from build123d import *

# Parameters (mm, degrees)
SKETCH4_R             = 2.54
SKETCH4_R_2           = 1.8161
BOSS_EXTRUDE1_DEPTH   = 2.38125
BOSS_EXTRUDE1_2_DEPTH = 2.38125
SKETCH5_R             = 1.7907
BOSS_EXTRUDE2_DEPTH   = 1.27


with BuildPart() as part:
    # Sketch4 → Boss-Extrude1 (new, symmetric)
    with BuildSketch(Plane.XY):
        with Locations(Location((-4.7625, 0, 0), (0, 0, 180))):
            Circle(SKETCH4_R)
        with Locations(Location((-4.7625, 0, 0), (0, 0, 180))):
            Circle(SKETCH4_R_2, mode=Mode.SUBTRACT)
    extrude(amount=BOSS_EXTRUDE1_DEPTH, both=True)


with BuildPart() as body_2:
    # Sketch4 → Boss-Extrude1 2 (new, symmetric)
    with BuildSketch(Plane.XY):
        with Locations(Location((4.7625, 0, 0), (0, 0, 180))):
            Circle(SKETCH4_R)
        with Locations(Location((4.7625, 0, 0), (0, 0, 180))):
            Circle(SKETCH4_R_2, mode=Mode.SUBTRACT)
    extrude(amount=BOSS_EXTRUDE1_2_DEPTH, both=True)


with BuildPart() as body_3:
    # Sketch5 → Boss-Extrude2 (new body)
    with BuildSketch(Plane.XY.offset(2.38125)):
        with BuildLine():
            ThreePointArc((-3.562267566, 4.240307738), (-9.1694, 0), (-3.562267566, -4.240307738))
            ThreePointArc((-3.562267566, -4.240307738), (0, -3.745865), (3.562267566, -4.240307738))
            ThreePointArc((3.562267566, -4.240307738), (9.1694, 0), (3.562267566, 4.240307738))
            ThreePointArc((3.562267566, 4.240307738), (0, 3.745865), (-3.562267566, 4.240307738))
        make_face()
        with Locations((-4.7625, 0)):
            Circle(SKETCH5_R, mode=Mode.SUBTRACT)
        with Locations((4.7625, 0)):
            Circle(SKETCH5_R, mode=Mode.SUBTRACT)
    extrude(amount=BOSS_EXTRUDE2_DEPTH)


with BuildPart() as body_4:
    # Mirror3: mirrored copy
    add(body_3.part.mirror(Plane.XY))

    # Combine2: union body 3, body 2, part
    add(body_3.part)
    add(body_2.part)
    add(part.part)


solid = body_4.part
For this review, take the finished solid that the model builds, in its own axes (mm). A direction names the side the tool comes from. Give positions to 0.01 mm unless a question says otherwise; leave off trailing zeros. Loops run counter-clockwise (first coordinate to the right, second up) from the corner with the lowest first, then second, coordinate; pieces in that order, holes last. Notation, with made-up numbers: M 64.5,32.25 L 87.5,32.25 A14 cw 87.5,38.25 Z; hole C -35.5,68 d6. An arc over 180 degrees is marked long. Answer as a JSON object with one key per item and string values. Group by question number.
Q1. Add section A-A on z = 0.75. Give the boundary of the cut face in (x, y), and give its area (3 significant figures).
Q2. Add section C-C on x = -1. Give the boundary of the cut face in (y, z).
Q3. Tool access review of faces 4 (the cylindrical face through (2.34, -0.76, 0.03)), 5 (the flat face through (0, 0, -3.651)): name each direction out of +Z, -Z, +X, -X, +Y, -Y from which nothing blocks a thin tool from reaching the whole face with its end or side.
Q4. Insertion check: P1, Ø1, axis at x = -6.5, z = 2, coming from the -Y side; P2, Ø1.5, axis at x = 5, z = 0, coming from the -Y side; P3, Ø4, axis at x = -5, y = -0.5, coming from the -Z side. Each pin has a flat end and moves straight along its axis. Give the tip position at first contact, or say it passes through.
Q5. For probe 1 along Z at (x, y) = (2.5, -1.5); probe 2 along X at (y, z) = (-1.25, 2.25); probe 3 along X at (y, z) = (1.5, -2.25), list the stretches that pass through material, from the lowest coordinate up. Write a range as [from, to].
Q6. Add section D-D on y = -2.25. Give the boundary of the cut face in (x, z).
Q7. Add section B-B on y = 0. Give the number of separate pieces and of enclosed holes in the cut face, and give its area (3 significant figures).
Q8. Mouldability with a two-part tool opening along Z and no side actions: class faces 1 (the flat face through (0, 0, -2.381)), 2 (the cylindrical face through (9.17, -0.11, -3.01)), 3 (the flat face through (0, 0, 3.651)) as +Z half, -Z half, draft (parallel to the pull), parting line (faces both ways), or undercut.
Checked values:
{
 "1": {"outline": "C -4.76,0 d5.08; C 4.76,0 d5.08; hole C -4.76,0 d3.63; hole C 4.76,0 d3.63", "area": "19.8 mm²"},
 "2": {"outline": "M -3.78,-3.65 L 3.78,-3.65 L 3.78,-2.38 L -3.78,-2.38 Z; M -3.78,2.38 L 3.78,2.38 L 3.78,3.65 L -3.78,3.65 Z"},
 "3": {"face 4": "none", "face 5": "-Z, +X, -X, +Y, -Y"},
 "4": {"P1": "y = -4.17", "P2": "y = -2.54", "P3": "z = -3.65"},
 "5": {"probe 1": "[-3.65, -2.38], [2.38, 3.65]", "probe 2": "[-6.97, -6.08], [-3.45, -2.55], [2.55, 3.45], [6.08, 6.97]", "probe 3": "[-6.81, -5.79], [-3.74, -2.71], [2.71, 3.74], [5.79, 6.81]"},
 "6": {"outline": "M -8.55,-3.65 L 8.55,-3.65 L 8.55,-2.38 L 5.94,-2.38 L 5.94,2.38 L 8.55,2.38 L 8.55,3.65 L -8.55,3.65 L -8.55,2.38 L -5.94,2.38 L -5.94,-2.38 L -8.55,-2.38 Z; hole M -3.58,-2.38 L 3.58,-2.38 L 3.58,2.38 L -3.58,2.38 Z"},
 "7": {"separate pieces": "3", "enclosed holes": "1", "area": "42.2 mm²"},
 "8": {"face 1": "undercut", "face 2": "draft", "face 3": "+Z half"}
}
